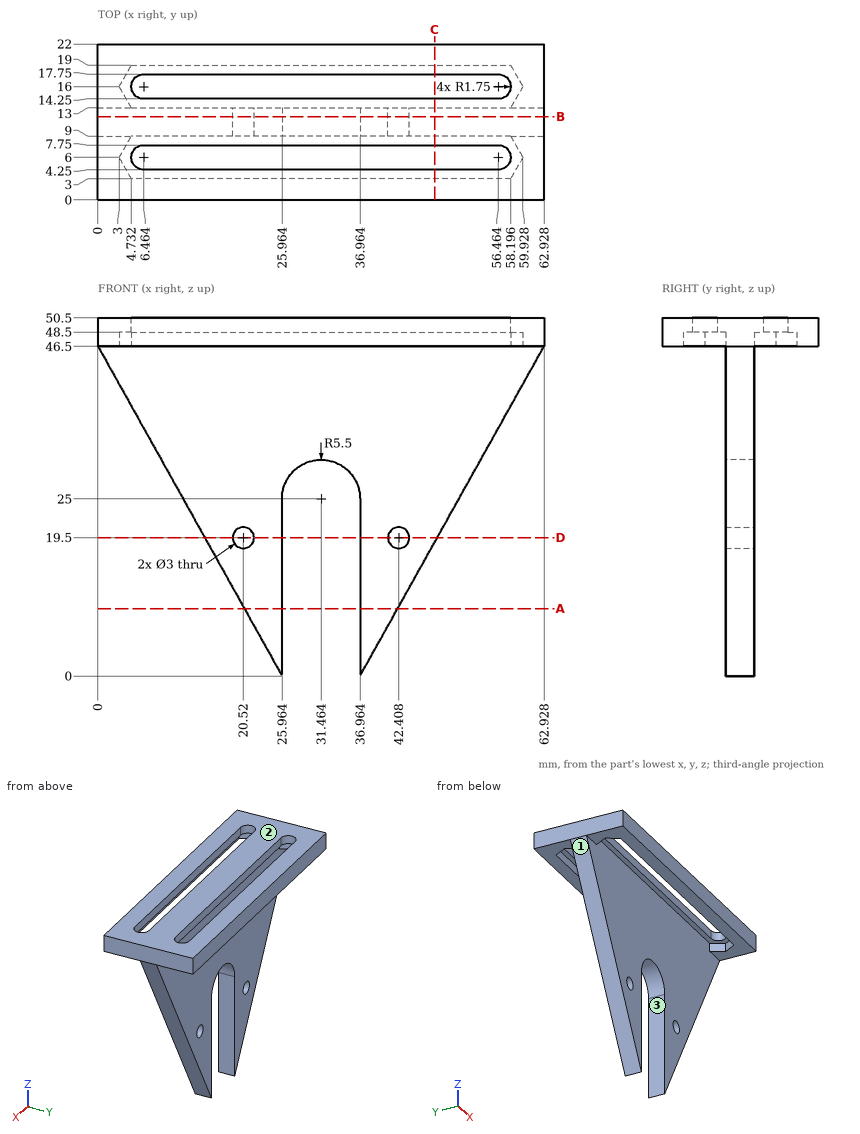
Job drawing, mm, ordinate dimensions from the low corner. One solid piece. Give positions to 0.01 mm unless a question says otherwise; leave off trailing zeros. Write each loop counter-clockwise with the first axis right and the second up, starting at its lowest first coordinate (ties: lowest second). Pieces come first, ordered by that corner, then holes. Notation, with made-up numbers: M 74,-26.5 L 91,-26.5 A20 cw 91,3.5 Z; hole C 9.25,61.25 d10. An arc over 180 degrees is marked long. Put each result on its own line as item: value. Start each with the question number.
(1) Probe L1, parallel to Y at x = 10.5, z = 47; L2, parallel to Y at x = 49.5, z = 25; L3, parallel to Z at x = 17.5, y = 2.75. List the from-to ranges inside material, lowest first.
(2) Band-saw the part on C-C, the plane x = 47.5. Write the cut outline in (y, z).
(3) Band-saw the part on A-A, the plane z = 9.5. Write the cut outline in (x, y).
(4) Band-saw the part on D-D, the plane z = 19.5. Write the cut outline in (x, y).
(5) Mould opens along X. For the marked faces 1, 2 and 3 say: +X half, -X half, draft (parallel to the pull), parting line (faces both ways), or undercut.
(6) Band-saw the part on B-B, the plane y = 11.75. Write the cut outline in (x, z).
(7) Flat gauge pins, fed straight in: pin 1 Ø0.6 at (x, z) = (25.5, 48) entering from -Y; pin 2 Ø12 at (y, z) = (12.5, 26.5) entering from +X; pin 3 Ø1.5 at (x, z) = (24, 18) entering from +Y; pin 4 Ø10 at (x, y) = (36, 19.5) entering from -Z. Where does each tip first touch, or does it go through?
Response values:
1. L1: y = 0 to 3, 9 to 13, 19 to 22
1. L2: y = 9 to 13
1. L3: z = 46.5 to 50.5
2. outline: M 0,46.5 L 3,46.5 L 3,48.5 L 4.25,48.5 L 4.25,50.5 L 0,50.5 Z; M 7.75,48.5 L 9,48.5 L 9,18.87 L 13,18.87 L 13,48.5 L 14.25,48.5 L 14.25,50.5 L 7.75,50.5 Z; M 17.75,48.5 L 19,48.5 L 19,46.5 L 22,46.5 L 22,50.5 L 17.75,50.5 Z
3. outline: M 20.66,9 L 25.96,9 L 25.96,13 L 20.66,13 Z; M 36.96,9 L 42.27,9 L 42.27,13 L 36.96,13 Z
4. outline: M 15.08,9 L 19.02,9 L 19.02,13 L 15.08,13 Z; M 22.02,9 L 25.96,9 L 25.96,13 L 22.02,13 Z; M 36.96,9 L 40.91,9 L 40.91,13 L 36.96,13 Z; M 43.91,9 L 47.85,9 L 47.85,13 L 43.91,13 Z
5. face 1: -X half
5. face 2: draft
5. face 3: undercut
6. outline: M 0,46.5 L 25.96,0 L 25.96,25 A5.5 cw 36.96,25 L 36.96,0 L 62.93,46.5 L 62.93,50.5 L 0,50.5 Z; hole C 20.52,19.5 d3; hole C 42.41,19.5 d3
7. pin 1: stops at y = 0
7. pin 2: stops at x = 55.11
7. pin 3: stops at y = 13
7. pin 4: stops at z = 46.5
